Autodesk Fusion 360 part; units mm, degrees
sketch "windowThroughHoles" plane through (0, 0, 0) normal (0, 0, 1) x (1, 0, 0)
  line L0 (0, 0) -> (14, 0)
  line L1 (0, 5) -> (5, 18)
  circle A0 centre (7, 15.5) radius 1
  circle A1 centre (2.5, 2.5) radius 1
  circle A2 centre (11.5, 2.5) radius 1
  line L2 (14, 18) -> (0, 18)
  line L3 (0, 18) -> (0, 0)
  line L4 (5, 18) -> (9, 18)
  line L5 (0, 0) -> (0, 5)
  line L6 (14, 5) -> (9, 18)
  line L7 (0, 0) -> (14, 0)
  line L8 (14, 0) -> (14, 5)
  line L9 (14, 0) -> (14, 18)
  dimension "d1" = 13
  dimension "d2" = 4.5
  dimension "d3" = 13
  dimension "d4" = 4.5
  dimension "d5" = 18
  dimension "d6" = 14
  dimension "d7" = 13.9284
  dimension "d8" = 13.9284
  dimension "d9" = 4
  dimension "d10" = 2
extrude "Extrude1" add sketch "windowThroughHoles" along normal blind 1.7526 contours L0 L1 L2 L3 L4 L5 L6 L7 L8 L9
Geometry: final body of the model. Coordinates: model frame, mm. Round coordinates to 2 decimals unless told otherwise and drop trailing zeros. Order: outer loops, then holes, each group sorted by start corner. A loop starts at its lowest first (then second) coordinate and runs counter-clockwise, first axis right, second up. Notation, with made-up numbers: M 42.25,19.25 L 72.25,19.25 A28 ccw 72.25,57.25 Z; hole C 16.25,-1 d11. An arc over 180 degrees is marked long. One line per item, written item: value.
(1) Pull-direction query (X, two-part tool) for faces 1 (the flat face through (7, 18, 1)), 2 (the cylindrical face through (6.783, 16.476, 0.864)), 3 (the flat face through (14, 2, 1)); classes: pulls with the +X half, pulls with the -X half, needs draft (parallel to the pull), parting line crosses it, or undercut.
Result sheet:
face 1: needs draft
face 2: undercut
face 3: pulls with the +X half
(2) Line query: probe 1 along Y at (x, z) = (7, 1); probe 2 along X at (y, z) = (3.25, 0.8); probe 3 along X at (y, z) = (3, 0.35). Output: solid intervals per line, ascending. Write a range as [from, to].
Result sheet:
probe 1: [0, 14.5], [16.5, 18]
probe 2: [0, 1.84], [3.16, 10.84], [12.16, 14]
probe 3: [0, 1.63], [3.37, 10.63], [12.37, 14]
(3) Cut plane A-A (z = 0.25). Return the cut outline in (x, y).
Result sheet:
outline: M 0,0 L 14,0 L 14,5 L 9,18 L 5,18 L 0,5 Z; hole C 2.5,2.5 d2; hole C 7,15.5 d2; hole C 11.5,2.5 d2
(4) Cut plane B-B (x = 2.5). Return the cut outline in (y, z).
Result sheet:
outline: M 0,0 L 1.5,0 L 1.5,1.75 L 0,1.75 Z; M 3.5,0 L 11.5,0 L 11.5,1.75 L 3.5,1.75 Z
(5) Cut plane C-C (y = 2.5). Return the cut outline in (x, z).
Result sheet:
outline: M 0,0 L 1.5,0 L 1.5,1.75 L 0,1.75 Z; M 3.5,0 L 10.5,0 L 10.5,1.75 L 3.5,1.75 Z; M 12.5,0 L 14,0 L 14,1.75 L 12.5,1.75 Z
(6) Cut plane D-D (x = 7). Return the cut outline in (y, z).
Result sheet:
outline: M 0,0 L 14.5,0 L 14.5,1.75 L 0,1.75 Z; M 16.5,0 L 18,0 L 18,1.75 L 16.5,1.75 Z
